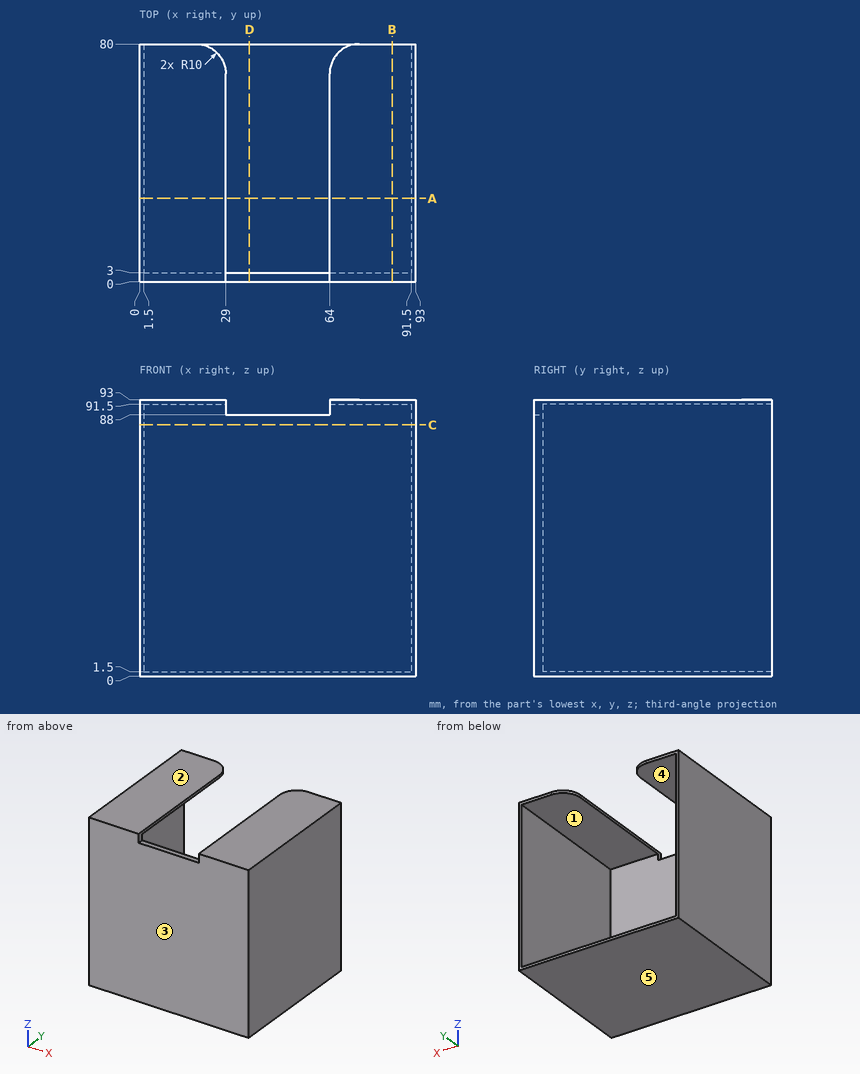
Drawing for the job (mm, zero at the part's lowest x, y, z). A direction names the side the tool comes from. Coordinates: 2 decimals unless noted, no trailing zeros. Order: outer loops, then holes, each group sorted by start corner. A loop starts at its lowest first (then second) coordinate and runs counter-clockwise, first axis right, second up. Notation, with made-up numbers: (-27, 74.25) -> (31, 74.25) arc R15 ccw to (31, 89.25) -> close; hole circle Ø3 at (77.25, 33.25). An arc over 180 degrees is marked (long way). Return JSON: item names as keys, results as strings.
Item 1: Mould opens along Z. For the marked faces 3, 4 and 5 say: pulls with the +Z half, pulls with the -Z half, needs draft (parallel to the pull), parting line crosses it, or undercut.
Model answer:
{"face 3": "needs draft", "face 4": "undercut", "face 5": "pulls with the -Z half"}
Item 2: 3-axis set-ups, long thin cutter, end or side, ignore diameter. For the marked faces 1 and 2: which of +Z, -Z, +X, -X, +Y, -Y reach the whole face in a straight line?
Model answer:
{"face 1": "+Y", "face 2": "+Z, +X, -X, +Y, -Y"}
Item 3: Slice it at C-C (z = 84.5). Write the cut outline in (x, y).
Model answer:
{"outline": "(0, 0) -> (93, 0) -> (93, 80) -> (91.5, 80) -> (91.5, 3) -> (1.5, 3) -> (1.5, 80) -> (0, 80) -> close"}
Item 4: Slice it at A-A (y = 28). Write the cut outline in (x, z), then the cut area to 4 significant figures.
Model answer:
{"outline": "(0, 0) -> (93, 0) -> (93, 93) -> (64, 93) -> (64, 91.5) -> (91.5, 91.5) -> (91.5, 1.5) -> (1.5, 1.5) -> (1.5, 91.5) -> (29, 91.5) -> (29, 93) -> (0, 93) -> close", "area": "496.5 mm²"}
Item 5: Slice it at B-B (x = 85). Write the cut outline in (y, z).
Model answer:
{"outline": "(0, 0) -> (80, 0) -> (80, 1.5) -> (3, 1.5) -> (3, 91.5) -> (80, 91.5) -> (80, 93) -> (0, 93) -> close"}
Item 6: Slice it at D-D (x = 37). Write the cut outline in (y, z).
Model answer:
{"outline": "(0, 0) -> (80, 0) -> (80, 1.5) -> (3, 1.5) -> (3, 88) -> (0, 88) -> close"}
Item 7: Pin check, flat tips, straight feed: P1, Ø5, axis at x = 61.5, z = 16.5, coming from the +Y side; P2, Ø1.5, axis at x = 40.5, y = 2, coming from the +Z side. Stop position of each tip, or through.
Model answer:
{"P1": "stops at y = 3", "P2": "stops at z = 88"}
Item 8: Wall check: line 1 along X through (y, z) = (76.5, 23); line 2 along Z through (x, y) = (44.5, 20.5). Give the ranges that are in metal, low to high. Write a range as from..to.
Model answer:
{"line 1": "x = 0..1.5, 91.5..93", "line 2": "z = 0..1.5"}
